Source: CAD feature listing. Evaluate the final solid. Frame: model axes, mm. Face numbers are marked on the shaded views. A direction names the side the tool comes from. Coordinates: 2 decimals unless noted, no trailing zeros. Loops run counter-clockwise (first coordinate to the right, second up) from the corner with the lowest first, then second, coordinate; pieces in that order, holes last.
from build123d import *

# Parameters (mm, degrees)
SKETCH1_R               = 4
BOSS_EXTRUDE2_DEPTH     = 13
SKETCH2_R               = 3.175
BOSS_EXTRUDE3_DEPTH     = 6
SKETCH3_R               = 2.775
BOSS_EXTRUDE4_DEPTH     = 4
CUT_EXTRUDE1_DEPTH      = 24.685438565
CUT_EXTRUDE1_DEPTH_BACK = 24.685438565
SKETCH4_R               = 1.5


with BuildPart() as part:
    # Sketch1 → Boss-Extrude2 (new body)
    with BuildSketch(Plane.XY):
        with Locations(Location((0, 0, 0), (0, 0, 180))):
            Circle(SKETCH1_R)
    extrude(amount=BOSS_EXTRUDE2_DEPTH)

    # Sketch2 → Boss-Extrude3 (add)
    with BuildSketch(Plane.XY.offset(13)):
        Circle(SKETCH2_R)
    extrude(amount=BOSS_EXTRUDE3_DEPTH)

    # Sketch3 → Boss-Extrude4 (add)
    with BuildSketch(Plane.XY.offset(19)):
        Circle(SKETCH3_R)
    extrude(amount=BOSS_EXTRUDE4_DEPTH)

    # Sketch4 → Cut-Extrude1 (cut, two sides: drawn at the far end of the back side and taken through both)
    with BuildSketch(Plane(origin=(0, 0, 0), x_dir=(1, 0, 0), z_dir=(0, 1, 0)).offset(-CUT_EXTRUDE1_DEPTH_BACK)):
        with Locations(Location((0, -16.55, 0), (0, 0, 270))):
            Circle(SKETCH4_R)
    extrude(amount=CUT_EXTRUDE1_DEPTH + CUT_EXTRUDE1_DEPTH_BACK, mode=Mode.SUBTRACT)


solid = part.part
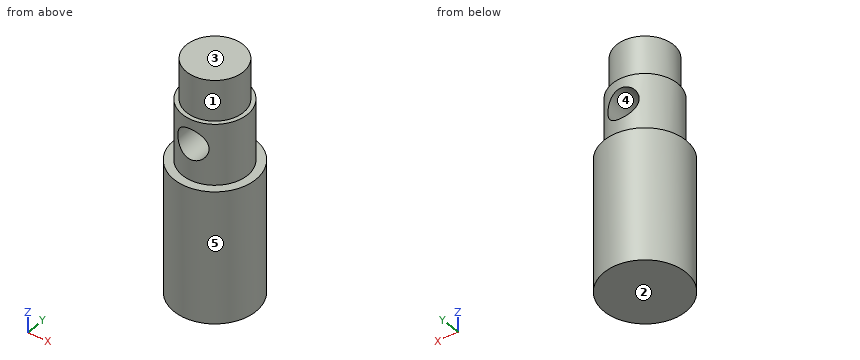
Q1. Section B-B, the plane x = 0. Return the cut outline in (y, z) (3 decimals).
Q2. Access query for the marked faces 1 and 2. Directions: +Z, -Z, +X, -X, +Y, -Y. A direction counts if a zero-diameter tool reaches every point of the face in a straight line with its end or side. Return the directions, or none.
Q3. Section C-C, the plane z = 5.75. Return the cut outline in (x, y), plus the area to 3 significant figures.
Q4. Section A-A, the plane y = 0. Return the cut outline in (x, z) (3 decimals), plus the area to 3 significant figures.
Q5. Draft query along Z for the marked faces 3, 4 and 5. Return one class per face: +Z half, -Z half, draft (parallel to the pull), parting line (faces both ways), or undercut.
Q6. Line query: line 1 along Z through (x, y) = (0, -0.5); line 2 along X through (y, z) = (1.5, 16.55); line 3 along Z through (x, y) = (1.5, -3.25). Output: solid intervals per line, ascending.
Q7. Section D-D, the plane y = 1.5. Return the cut outline in (x, z).
Q8. Contact query for a flat-ended pin moving along its axis: pin 1 Ø3 at (y, z) = (3, 12.5) entering from +X. Output: stop coordinate, or through.
Derived:
1. outline: (-4, 0) - (4, 0) - (4, 13) - (3.175, 13) - (3.175, 15.05) - (-3.175, 15.05) - (-3.175, 13) - (-4, 13) - close; (-3.175, 18.05) - (3.175, 18.05) - (3.175, 19) - (2.775, 19) - (2.775, 23) - (-2.775, 23) - (-2.775, 19) - (-3.175, 19) - close
2. face 1: +Z
2. face 2: -Z, +X, -X, +Y, -Y
3. outline: circle Ø8 at (0, 0)
3. area: 50.3 mm2
4. outline: (-4, 0) - (4, 0) - (4, 13) - (3.175, 13) - (3.175, 19) - (2.775, 19) - (2.775, 23) - (-2.775, 23) - (-2.775, 19) - (-3.175, 19) - (-3.175, 13) - (-4, 13) - close; hole circle Ø3 at (0, 16.55)
4. area: 157 mm2
5. face 3: +Z half
5. face 4: undercut
5. face 5: draft
6. line 1: z = 0 to 15.05, 18.05 to 23
6. line 2: x = -2.8 to -1.5, 1.5 to 2.8
6. line 3: z = 0 to 13
7. outline: (-3.71, 0) - (3.71, 0) - (3.71, 13) - (2.8, 13) - (2.8, 19) - (2.33, 19) - (2.33, 23) - (-2.33, 23) - (-2.33, 19) - (-2.8, 19) - (-2.8, 13) - (-3.71, 13) - close; hole circle Ø3 at (0, 16.55)
8. pin 1: stops at x = 3.71
